CAD build for the part. Positions are in the model's coordinates, mm. Face numbers are marked on the shaded views. Give positions to 0.01 mm unless a question says otherwise; leave off trailing zeros. Write each loop counter-clockwise with the first axis right and the second up, starting at its lowest first coordinate (ties: lowest second). Pieces come first, ordered by that corner, then holes. Notation, with made-up numbers: (-30.5, 49.5) -> (13.5, 49.5) arc R15 ccw to (13.5, 60.5) -> close; hole circle Ø5 at (36, -30). An arc over 180 degrees is marked (long way). Use one line per item in the form item = value. Start each with the question number.
Autodesk Inventor part; units mm, degrees
ref_plane "YZ Plane" through (0, 0, 0) normal (1, 0, 0) x (0, 1, 0)
ref_plane "XZ Plane" through (0, 0, 0) normal (0, 1, 0) x (-1, 0, 0)
ref_plane "XY Plane" through (0, 0, 0) normal (0, 0, 1) x (1, 0, 0)
sketch "スケッチ1" plane through (0, 0, 0) normal (0, 0, 1) x (1, 0, 0)
  line L0 (-15, 19.05) -> (15, 19.05)
  line L1 (15, 19.05) -> (15, -13.95)
  line L2 (15, -13.95) -> (-15, -13.95)
  line L3 (-15, -13.95) -> (-15, 19.05)
  point P0 (0, 0)
  dimension "d0" = 30
  dimension "d1" = 33
  dimension "d2" = 19.05
  dimension "d3" = 15
extrude "押し出し1" add sketch "スケッチ1" along normal blind 5
sketch "スケッチ2" plane through (0, 0, 0) normal (0, 0, 1) x (1, 0, 0)
  circle A0 centre (0, 0) radius 6
  dimension "d6" = 12
extrude "押し出し2" cut sketch "スケッチ2" along normal blind 5
fillet "フィレット1" radius 2 4 edges at (15, 19.05, 2.5) (15, -13.95, 2.5) (-15, -13.95, 2.5) (-15, 19.05, 2.5)
properties part number "HbSensorCushion01" material "ゴム"
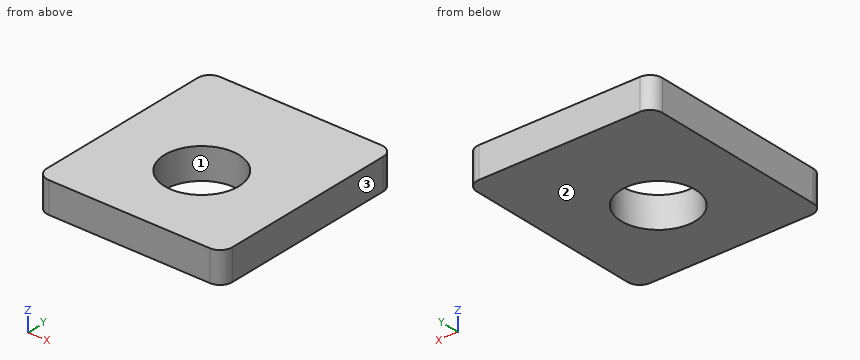
1) Wall check: line 1 along Y through (x, z) = (0, 2.35); line 2 along X through (y, z) = (0.5, 3.1); line 3 along Y through (x, z) = (-3.25, 0.65). Give the ranges that are in metal, low to high. Write a range as from..to.
2) Pin check, flat tip, straight feed: pin 1 (7 mm diameter, centred on x = 0, y = 0, fed in from -Z). Stop position of the tip, or through.
3) Cut at C-C (z = 2.8). Give the cut face in (x, y).
4) Two-plate mould, pull along X, no slides. Class the marked faces 1, 2 and 3: released by +X, released by -X, zero draft, split by the parting line, or undercut.
5) Cut at B-B (y = 0). Give the cut face in (x, z), and give its area (3 significant figures).
6) Cut at A-A (x = 0). Give the cut face in (y, z), and give its area (3 significant figures).
Final values:
q1.line_1 = -13.95..-6, 6..19.05
q1.line_2 = -15..-5.98, 5.98..15
q1.line_3 = -13.95..-5.04, 5.04..19.05
q2.pin_1 = through
q3.outline = (-15, -11.95) arc R2 ccw to (-13, -13.95) -> (13, -13.95) arc R2 ccw to (15, -11.95) -> (15, 17.05) arc R2 ccw to (13, 19.05) -> (-13, 19.05) arc R2 ccw to (-15, 17.05) -> close; hole circle Ø12 at (0, 0)
q4.face_1 = undercut
q4.face_2 = zero draft
q4.face_3 = released by +X
q5.outline = (-15, 0) -> (-6, 0) -> (-6, 5) -> (-15, 5) -> close; (6, 0) -> (15, 0) -> (15, 5) -> (6, 5) -> close
q5.area = 90.0 mm^2
q6.outline = (-13.95, 0) -> (-6, 0) -> (-6, 5) -> (-13.95, 5) -> close; (6, 0) -> (19.05, 0) -> (19.05, 5) -> (6, 5) -> close
q6.area = 105 mm^2
